Can you work these out from the drawing? Everything is in mm from the part's minimum corner. A direction names the side the tool comes from. Coordinates: 2 decimals unless noted, no trailing zeros. Order: outer loops, then holes, each group sorted by start corner. A loop starts at its lowest first (then second) coordinate and runs counter-clockwise, first axis right, second up. Notation, with made-up numbers: (61.5, -17) - (106.5, -17) arc R14 ccw to (106.5, 2) - close; hole circle Ø11 at (-25, 84). An arc over 180 degrees is marked (long way). Use a Markdown table: item, result. Add a question column.
(1) On a 3-axis mill with a long thin cutter (end or side, diameter ignored), from which of +Z, -Z, +X, -X, +Y, -Y can I reach the whole of each face in a straight line? I mean the marked faces 4 and 5. Say none if no direction works.
(2) If I drill on L1, parallel to Z at x = 16, y = 3; L2, parallel to Y at x = 10.5, z = 42; L3, parallel to X at y = 2, z = 47.5, over which ranges is the centre line in solid material (lowest first)? Write a range as [from, to].
(3) I want a section at D-D (z = 20.5). List the corners of the cut face in (x, y) for me (1 decimal).
(4) For pin 1 Ø1.1 at (x, y) = (2, 1.5) entering from +Z; pin 2 Ø3.5 at (y, z) = (4.5, 35) entering from +X; pin 3 Ø3 at (x, y) = (5.5, 2.5) entering from -Z, each with a flat end and sliding along its axis, tell me the tip position at first contact or that it passes through.
(5) I want a section at A-A (x = 15.25). List the corners of the cut face in (y, z) for me, and give its area (3 significant figures).
(6) We'd pull the mould along Z, two halves only. Please class the marked faces 1, 2 and 3: pulls with the +Z half, pulls with the -Z half, needs draft (parallel to the pull), parting line crosses it, or undercut.
(7) I want a section at B-B (y = 1.75). List the corners of the cut face in (x, z) for me, and give its area (3 significant figures).
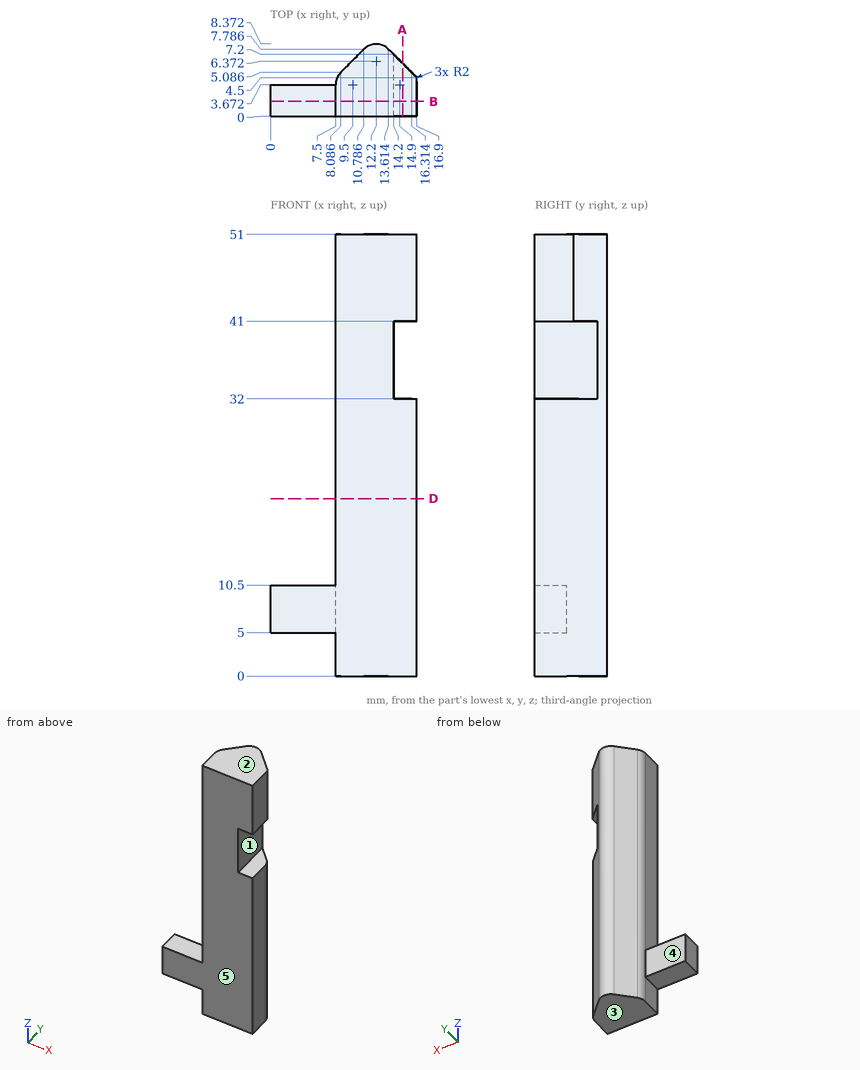
Answers follow:
| question | item | result |
|---|---|---|
| 1 | face 4 | +Z, -Z, -X, +Y |
| 1 | face 5 | +Z, -Z, +X, -X, -Y |
| 2 | L1 | z = [0, 32], [41, 51] |
| 2 | L2 | y = [0, 7.5] |
| 2 | L3 | x = [7.5, 16.9] |
| 3 | outline | (7.5, 0) - (16.9, 0) - (16.9, 3.7) arc R2 ccw to (16.3, 5.1) - (13.6, 7.8) arc R2 ccw to (10.8, 7.8) - (8.1, 5.1) arc R2 ccw to (7.5, 3.7) - close |
| 4 | pin 1 | stops at z = 10.5 |
| 4 | pin 2 | stops at x = 14.2 |
| 4 | pin 3 | stops at z = 5 |
| 5 | outline | (0, 0) - (6.15, 0) - (6.15, 32) - (0, 32) - close; (0, 41) - (6.15, 41) - (6.15, 51) - (0, 51) - close |
| 5 | area | 258 mm² |
| 6 | face 1 | undercut |
| 6 | face 2 | pulls with the +Z half |
| 6 | face 3 | pulls with the -Z half |
| 7 | outline | (0, 5) - (7.5, 5) - (7.5, 0) - (16.9, 0) - (16.9, 32) - (14.2, 32) - (14.2, 41) - (16.9, 41) - (16.9, 51) - (7.5, 51) - (7.5, 10.5) - (0, 10.5) - close |
| 7 | area | 496 mm² |
